from build123d import *

# Parameters (mm, degrees)
SKETCH001_W      = 20
SKETCH001_H      = 15
SKETCH001_W_2    = 10
SKETCH001_H_2    = 5
EXTRUDE001_DEPTH = 2.5
SKETCH002_W      = 90
SKETCH002_H      = 30
EXTRUDE002_DEPTH = 40
SKETCH_W         = 100
SKETCH_H         = 40
EXTRUDE_DEPTH    = 7.5
FILLET_R         = 10
FILLET001_R      = 1
FILLET002_R      = 1
FILLET003_R      = 1
FILLET004_R      = 1


with BuildPart() as extrude001:
    # Sketch001 (on Sketch) → Extrude001 (new body, symmetric)
    with BuildSketch(Plane.XY):
        with Locations((-60, 0)):
            Rectangle(SKETCH001_W, SKETCH001_H)
        with Locations((-60, 0)):
            Rectangle(SKETCH001_W_2, SKETCH001_H_2, mode=Mode.SUBTRACT)
        with Locations((60, 0)):
            Rectangle(SKETCH001_W, SKETCH001_H)
        with Locations((60, 0)):
            Rectangle(SKETCH001_W_2, SKETCH001_H_2, mode=Mode.SUBTRACT)
    extrude(amount=EXTRUDE001_DEPTH, both=True)


with BuildPart() as extrude002:
    # Sketch002 (on Face6 of Extrude) → Extrude002 (new body)
    with BuildSketch(Plane.XY.offset(7.5)):
        Rectangle(SKETCH002_W, SKETCH002_H)
    extrude(amount=EXTRUDE002_DEPTH)


with BuildPart() as extrude002_1:
    # Extrude002 placement: moved
    add(extrude002.part.moved(Location((0, 0, -28))))


with BuildPart() as fillet004:
    # Sketch → Extrude (new body, symmetric)
    with BuildSketch(Plane.XY):
        Rectangle(SKETCH_W, SKETCH_H)
    extrude(amount=EXTRUDE_DEPTH, both=True)

    # Cut: cut Extrude002
    add(extrude002_1.part, mode=Mode.SUBTRACT)

    # Fillet
    fillet_edges = [fillet004.edges().sort_by_distance(p)[0] for p in [
        (45, -15, 0),
        (-45, -15, 0),
        (45, 15, 0),
        (-45, 15, 0),
    ]]
    fillet(fillet_edges, radius=FILLET_R)

    # Fusion: union Extrude001
    add(extrude001.part)

    # Fillet001
    fillet001_edges = [fillet004.edges().sort_by_distance(p)[0] for p in [
        (0, -20, -7.5),
        (0, 20, -7.5),
        (0, -20, 7.5),
        (0, 20, 7.5),
    ]]
    fillet(fillet001_edges, radius=FILLET001_R)

    # Fillet002
    fillet002_edges = [fillet004.edges().sort_by_distance(p)[0] for p in [
        (0, -15, -7.5),
        (42.071068, -12.071068, -7.5),
        (-42.071068, -12.071068, -7.5),
        (45, 0, -7.5),
        (-45, 0, -7.5),
        (42.071068, 12.071068, -7.5),
        (-42.071068, 12.071068, -7.5),
        (0, 15, -7.5),
        (0, -15, 7.5),
        (42.071068, -12.071068, 7.5),
        (-42.071068, -12.071068, 7.5),
        (45, 0, 7.5),
        (-45, 0, 7.5),
        (42.071068, 12.071068, 7.5),
        (-42.071068, 12.071068, 7.5),
        (0, 15, 7.5),
    ]]
    fillet(fillet002_edges, radius=FILLET002_R)

    # Fillet003
    fillet003_edges = [fillet004.edges().sort_by_distance(p)[0] for p in [
        (70, 7.5, 0),
        (60, 7.5, -2.5),
        (60, 7.5, 2.5),
        (60, -7.5, 2.5),
        (70, 0, 2.5),
        (70, -7.5, 0),
        (60, -7.5, -2.5),
        (70, 0, -2.5),
    ]]
    fillet(fillet003_edges, radius=FILLET003_R)

    # Fillet004
    fillet004_edges = [fillet004.edges().sort_by_distance(p)[0] for p in [
        (-70, 0, -2.5),
        (-60, -7.5, -2.5),
        (-60, 7.5, -2.5),
        (-70, 7.5, 0),
        (-60, 7.5, 2.5),
        (-70, 0, 2.5),
        (-60, -7.5, 2.5),
        (-70, -7.5, 0),
    ]]
    fillet(fillet004_edges, radius=FILLET004_R)


solid = fillet004.part
The model under review builds one solid part; all positions refer to its coordinate system, in mm. A direction names the side the tool comes from. Round coordinates to 2 decimals unless told otherwise and drop trailing zeros. Loops run counter-clockwise (first coordinate to the right, second up) from the corner with the lowest first, then second, coordinate; pieces in that order, holes last. Notation, with made-up numbers: M 42.5,-7.5 L 76.5,-7.5 A18 cw 76.5,14.5 Z; hole C 52,43 d6. An arc over 180 degrees is marked long. Answer as a JSON object with one key per item and string values.
Item 1: The part is to be moulded in two halves that separate along X. For faces 4 (the face through (50, 0, 3)), 5 (the face through (-60, 3, -2.5)), 6 (the face through (-60, -2.5, 0)), 7 (the face through (45, 0, 0)), say which applies: +X half, -X half, draft (parallel to the pull), parting line (faces both ways), or undercut.
Check sheet entries:
{"face 4": "+X half", "face 5": "draft", "face 6": "undercut", "face 7": "undercut"}
Item 2: Tool access review of faces 1 (the face through (-45, 0, 0)), 2 (the face through (59, 3, -2.5)), 3 (the face through (59, -7.5, 0)): name each direction out of +Z, -Z, +X, -X, +Y, -Y from which nothing blocks a thin tool from reaching the whole face with its end or side.
Check sheet entries:
{"face 1": "+Z, -Z", "face 2": "-Z, +X, +Y, -Y", "face 3": "+Z, -Z, +X, -Y"}
Item 3: We need section C-C, the plane z = -5.25. State the section outline as (x, y) points, and give its area (3 significant figures).
Check sheet entries:
{"outline": "M -50,-20 L 50,-20 L 50,20 L -50,20 Z; hole M -45,-5 A10 ccw -35,-15 L 35,-15 A10 ccw 45,-5 L 45,5 A10 ccw 35,15 L -35,15 A10 ccw -45,5 Z", "area": "1,390 mm2"}
Item 4: We need section B-B, the plane y = -0.5. State how many separate pieces and enclosed holes the cut face has, and give its area (3 significant figures).
Check sheet entries:
{"separate pieces": "4", "enclosed holes": "0", "area": "248 mm2"}
Item 5: We need section A-A, the plane x = 17. State the section outline as (y, z) points.
Check sheet entries:
{"outline": "M -20,-6.5 A1 ccw -19,-7.5 L -16,-7.5 A1 ccw -15,-6.5 L -15,6.5 A1 ccw -16,7.5 L -19,7.5 A1 ccw -20,6.5 Z; M 15,-6.5 A1 ccw 16,-7.5 L 19,-7.5 A1 ccw 20,-6.5 L 20,6.5 A1 ccw 19,7.5 L 16,7.5 A1 ccw 15,6.5 Z"}
Item 6: We need section D-D, the plane x = -53.5. State the section outline as (y, z) points.
Check sheet entries:
{"outline": "M -7.5,-1.5 A1 ccw -6.5,-2.5 L 6.5,-2.5 A1 ccw 7.5,-1.5 L 7.5,1.5 A1 ccw 6.5,2.5 L -6.5,2.5 A1 ccw -7.5,1.5 Z"}
Item 7: Clearance check with flat-ended pins moving along their axes: P1, Ø0.9, axis at x = -64, z = 0, coming from the -Y side; P2, Ø6.5, axis at x = 62.5, y = -1, coming from the +Z side; P3, Ø6.5, axis at x = 59.5, y = 0, coming from the -Z side. State where each tip first meets the part, or that it passes through.
Check sheet entries:
{"P1": "y = -7.5", "P2": "z = 2.5", "P3": "z = -2.5"}
Item 8: For line 1 along Y through (x, z) = (-13, -5.5); line 2 along X through (y, z) = (-3.5, -3.25); line 3 along X through (y, z) = (16.5, -5.5), list the stretches that pass through material, from the lowest coordinate up.
Check sheet entries:
{"line 1": "-20 to -15, 15 to 20", "line 2": "-50 to -45, 45 to 50", "line 3": "-50 to 50"}
